Geometry: final body of the model. Coordinates: model frame, mm. Face numbers are marked on the shaded views. A direction names the side the tool comes from. Coordinates: 2 decimals unless noted, no trailing zeros. Order: outer loops, then holes, each group sorted by start corner. A loop starts at its lowest first (then second) coordinate and runs counter-clockwise, first axis right, second up. Notation, with made-up numbers: (63.25, 12) - (118.25, 12) arc R7 cw to (118.25, 18) - close; hole circle Ø10 at (12, 37). An arc over 180 degrees is marked (long way). Use a Markdown table: item, result. Add a question column.
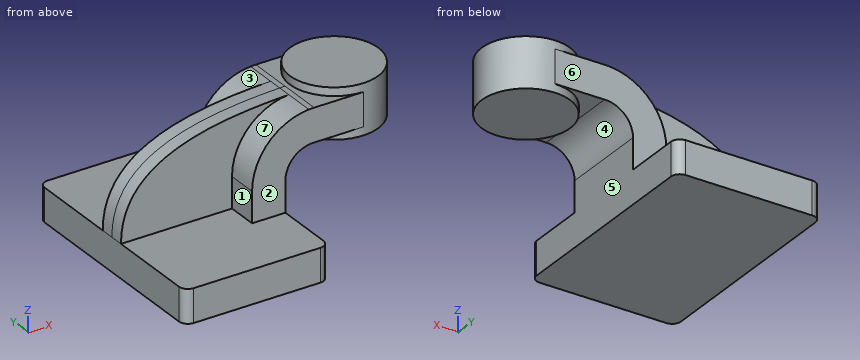
```python
from build123d import *

# Parameters (mm, degrees)
F1_DEPTH = 63.5
F0_W     = 25.5068594253
F0_H     = 19.05
F2_DEPTH = 25.4
F4_DEPTH = 7.9375
F5_R     = 5.08


with BuildPart() as f1:
    # F0 (on Front) → F1 (new body, symmetric)
    with BuildSketch(Plane.XZ):
        Polygon((22.225, 9.525), (-41.275, 9.525), (-41.275, -9.525), (41.275, -9.525), (41.275, 9.525), align=None)
    extrude(amount=F1_DEPTH, both=True)

    # F0 (on Front) → F2 (join, symmetric)
    with BuildSketch(Plane.XZ):
        with BuildLine():
            Line((22.225, 27.0052991994), (22.225, 9.525))
            Line((22.225, 9.525), (41.275, 9.525))
            Line((41.275, 9.525), (41.275, 27.0052991994))
            ThreePointArc((41.275, 27.0052991994), (46.0678396882, 38.3719762786), (57.5523351588, 42.8752))
            Line((57.5523351588, 42.8752), (60.325, 42.8752))
            Line((60.325, 42.8752), (60.325, 61.9252))
            Line((60.325, 61.9252), (57.7467856216, 61.9252))
            add(Edge.make_bspline(
                [(54.7118794678, 61.8450924432), (55.7241751025, 61.874777301), (56.735971204, 61.9013896481), (57.7467856217, 61.9252)],
                knots=[109.6921191668, 109.6921191668, 109.6921191668, 109.6921191668, 112.0316695749, 112.0316695749, 112.0316695749, 112.0316695749], degree=3))
            ThreePointArc((54.7118794678, 61.8450924432), (31.6068308095, 50.8234043446), (22.225, 27.0052991994))
        make_face()
        with Locations((73.0784297127, 52.4002)):
            Rectangle(F0_W, F0_H)
    extrude(amount=F2_DEPTH, both=True)

    # F0 (on Front) → F3 (revolve)
    with BuildSketch(Plane.XZ):
        Polygon((85.8318594253, 66.675), (85.8318594253, 61.9252), (85.8318594253, 42.8752), (85.8318594253, 38.1), (111.125, 38.1), (111.125, 66.675), align=None)
    revolve(axis=Axis((85.8318594253, 0, 52.3875), (0, 0, 1)))

    # F0 (on Front) → F4 (join, symmetric)
    with BuildSketch(Plane.XZ):
        with BuildLine():
            add(Edge.make_bspline(
                [(-41.275, 9.525), (-41.3111924675, 52.3071991607), (7.2494041966, 60.4532887264), (54.7118794678, 61.8450924432)],
                knots=[0, 0, 0, 0, 109.6921191668, 109.6921191668, 109.6921191668, 109.6921191668], degree=3))
            Line((-41.275, 9.525), (22.225, 9.525))
            Line((22.225, 9.525), (22.225, 27.0052991994))
            ThreePointArc((22.225, 27.0052991994), (31.6068308095, 50.8234043446), (54.7118794678, 61.8450924432))
        make_face()
    extrude(amount=F4_DEPTH, both=True)

    # F5
    f5_edges = [f1.edges().sort_by_distance(p)[0] for p in [
        (-41.275, -63.5, 0),
        (41.275, -63.5, 0),
        (41.275, 63.5, 0),
        (-41.275, 63.5, 0),
    ]]
    fillet(f5_edges, radius=F5_R)


solid = f1.part
```
1) Draft query along X for the marked faces 4, 5, 6 and 7. Return one class per face: released by +X, released by -X, zero draft, split by the parting line, or undercut.
2) First-contact query: pin 1 (1 mm diameter, centred on x = -9.5, y = -24, fed in from +Z) (3 decimals); pin 2 (15.5 mm diameter, centred on x = 16, z = 33, fed in from -Y); pin 3 (12 mm diameter, centred on x = -1, y = 8, fed in from +Z). Flat tips, straight axial feed; report the tip coordinate or a pass-through.
3) Line query: line 1 (X direction, y = 14.5, z = 26) (3 decimals); line 2 (Z direction, x = -21, y = 16) (3 decimals); line 3 (X direction, y = -11.5, z = 9) (3 decimals). Output: solid intervals per line, ascending. Write a range as from..to.
4) Section query A-A (z = -3). Return the cut outline in (x, y) (3 decimals), and give its area (3 significant figures).
5) Section query B-B (x = 78.5). Return the cut outline in (y, z) (3 decimals).
6) Access query for the marked faces 1, 2 and 3. Directions: +Z, -Z, +X, -X, +Y, -Y. A direction counts if a zero-diameter tool reaches every point of the face in a straight line with its end or side. Return the directions, or none.
7) Section query C-C (y = -46). Return the cut outline in (x, z) (3 decimals).
From the geometry:
| question | item | result |
|---|---|---|
| 1 | face 4 | undercut |
| 1 | face 5 | released by +X |
| 1 | face 6 | zero draft |
| 1 | face 7 | released by -X |
| 2 | pin 1 | stops at z = 9.525 |
| 2 | pin 2 | stops at y = -25.4 |
| 2 | pin 3 | stops at z = 56.33 |
| 3 | line 1 | x = 22.225..41.275 |
| 3 | line 2 | z = -9.525..9.525 |
| 3 | line 3 | x = -41.275..41.275 |
| 4 | outline | (-41.275, -58.42) arc R5.08 ccw to (-36.195, -63.5) - (36.195, -63.5) arc R5.08 ccw to (41.275, -58.42) - (41.275, 58.42) arc R5.08 ccw to (36.195, 63.5) - (-36.195, 63.5) arc R5.08 ccw to (-41.275, 58.42) - close |
| 4 | area | 10,500 mm^2 |
| 5 | outline | (-25.4, 42.875) - (-24.207, 42.875) - (-24.207, 38.1) - (24.207, 38.1) - (24.207, 42.875) - (25.4, 42.875) - (25.4, 61.925) - (24.207, 61.925) - (24.207, 66.675) - (-24.207, 66.675) - (-24.207, 61.925) - (-25.4, 61.925) - close |
| 6 | face 1 | +Z, -X, -Y |
| 6 | face 2 | +Z, +X, -X, -Y |
| 6 | face 3 | +Z, -X, +Y |
| 7 | outline | (-41.275, -9.525) - (41.275, -9.525) - (41.275, 9.525) - (-41.275, 9.525) - close |
